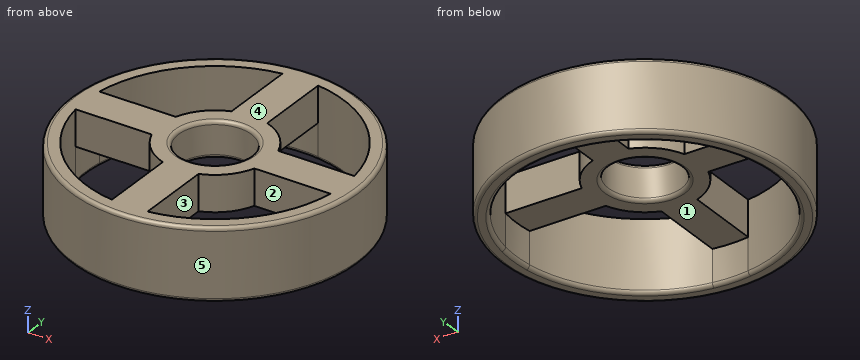
```python
from build123d import *

# Parameters (mm, degrees)
SKETCH2_R           = 20
BOSS_EXTRUDE1_DEPTH = 10
SKETCH4_R           = 5.1
CUT_EXTRUDE1_DEPTH  = 31
CUT_EXTRUDE2_START  = -5
SKETCH5_R           = 18
CUT_EXTRUDE2_DEPTH  = 5
FILLET1_R           = 0.5


with BuildPart() as part:
    # Sketch2 → Boss-Extrude1 (new body)
    with BuildSketch(Plane.XY):
        Circle(SKETCH2_R)
    extrude(amount=BOSS_EXTRUDE1_DEPTH)

    # Sketch4 → Cut-Extrude1 (cut, through all)
    with BuildSketch(Plane.XY.offset(10)):
        Circle(SKETCH4_R)
        with BuildLine():
            Line((-2.5, 17.82554347), (-2.5, 7.177046746))
            ThreePointArc((-2.5, 7.177046746), (-5.374011537, 5.374011537), (-7.177046746, 2.5))
            Line((-7.177046746, 2.5), (-17.82554347, 2.5))
            ThreePointArc((-17.82554347, 2.5), (-12.727922061, 12.727922061), (-2.5, 17.82554347))
        make_face()
        with BuildLine():
            Line((2.5, 17.82554347), (2.5, 7.177046746))
            ThreePointArc((2.5, 7.177046746), (5.374011537, 5.374011537), (7.177046746, 2.5))
            Line((7.177046746, 2.5), (17.82554347, 2.5))
            ThreePointArc((17.82554347, 2.5), (12.727922061, 12.727922061), (2.5, 17.82554347))
        make_face()
        with BuildLine():
            Line((7.177046746, -2.5), (17.82554347, -2.5))
            ThreePointArc((17.82554347, -2.5), (12.727922061, -12.727922061), (2.5, -17.82554347))
            Line((2.5, -17.82554347), (2.5, -7.177046746))
            ThreePointArc((2.5, -7.177046746), (5.374011537, -5.374011537), (7.177046746, -2.5))
        make_face()
        with BuildLine():
            Line((-7.177046746, -2.5), (-17.82554347, -2.5))
            ThreePointArc((-17.82554347, -2.5), (-12.727922061, -12.727922061), (-2.5, -17.82554347))
            Line((-2.5, -17.82554347), (-2.5, -7.177046746))
            ThreePointArc((-2.5, -7.177046746), (-5.374011537, -5.374011537), (-7.177046746, -2.5))
        make_face()
    extrude(amount=-CUT_EXTRUDE1_DEPTH, mode=Mode.SUBTRACT)

    # Sketch5 → Cut-Extrude2 (cut)
    with BuildSketch(Plane(origin=(0, 0, 0), x_dir=(-1, 0, 0), z_dir=(0, 0, -1)).offset(CUT_EXTRUDE2_START)):
        with Locations(Location((0, 0, 0), (0, 0, 172.016443854))):
            Circle(SKETCH5_R)
    extrude(amount=CUT_EXTRUDE2_DEPTH, mode=Mode.SUBTRACT)

    # Fillet1
    fillet1_edges = [part.edges().sort_by_distance(p)[0] for p in [
        (-20, 0, 0),
        (-18, 0, 0),
        (-5.1, 0, 10),
        (-20, 0, 10),
        (-5.1, 0, 5),
    ]]
    fillet(fillet1_edges, radius=FILLET1_R)


solid = part.part
```
Verification items for the finished model (mm, model axes). Face numbers are marked on the shaded views. A direction names the side the tool comes from. Coordinates: 2 decimals unless noted, no trailing zeros. Loops run counter-clockwise (first coordinate to the right, second up) from the corner with the lowest first, then second, coordinate; pieces in that order, holes last. Notation, with made-up numbers: (-33, 89) - (-4, 89) arc R35 ccw to (-4, 123) - close; hole circle Ø3 at (58, 61). An arc over 180 degrees is marked (long way). Return JSON: item names as keys, results as strings.
1. Section check A-A, the plane x = 0. Record the boundary of the cut face in (y, z).
Established:
{"outline": "(-20, 0.5) arc R0.5 ccw to (-19.5, 0) - (-18.5, 0) arc R0.5 ccw to (-18, 0.5) - (-18, 5) - (-5.6, 5) arc R0.5 ccw to (-5.1, 5.5) - (-5.1, 9.5) arc R0.5 ccw to (-5.6, 10) - (-19.5, 10) arc R0.5 ccw to (-20, 9.5) - close; (5.1, 5.5) arc R0.5 ccw to (5.6, 5) - (18, 5) - (18, 0.5) arc R0.5 ccw to (18.5, 0) - (19.5, 0) arc R0.5 ccw to (20, 0.5) - (20, 9.5) arc R0.5 ccw to (19.5, 10) - (5.6, 10) arc R0.5 ccw to (5.1, 9.5) - close"}
2. Go/stop test with flat-tipped pins: pin 1 (2.5 mm diameter, centred on x = 13, z = 8.5, fed in from +Y); pin 2 (6 mm diameter, centred on x = 10.5, z = 4, fed in from -Y); pin 3 (5.5 mm diameter, centred on y = 15, z = 7.5, fed in from -X); pin 4 (3 mm diameter, centred on x = 7.5, y = 7.5, fed in from -Z). Record where each tip stops, or that it passes through.
Established:
{"pin 1": "stops at y = 16.18", "pin 2": "stops at y = -18.54", "pin 3": "stops at x = -15.81", "pin 4": "passes through"}
3. Thickness scan on L1, parallel to Y at x = 0, z = 6.55; L2, parallel to X at y = 0.5, z = 4.75; L3, parallel to X at y = -6.5, z = 9.5. Record the ranges inside material, lowest first.
Established:
{"L1": "y = -20 to -5.1, 5.1 to 20", "L2": "x = -19.99 to -17.99, 17.99 to 19.99", "L3": "x = -18.91 to -16.79, -3.94 to 3.94, 16.79 to 18.91"}
4. Section check D-D, the plane y = -8.5. Count the separate pieces of the cut face and the enclosed holes in it, then the cut area to 3 significant figures.
Established:
{"separate pieces": "3", "enclosed holes": "0", "area": "69.4 mm2"}
5. Section check C-C, the plane z = 7. Record the boundary of the cut face in (x, y).
Established:
{"outline": "circle Ø40 at (0, 0); hole (-17.83, -2.5) arc R18 ccw to (-2.5, -17.83) - (-2.5, -7.18) arc R7.6 cw to (-7.18, -2.5) - close; hole (-17.83, 2.5) - (-7.18, 2.5) arc R7.6 cw to (-2.5, 7.18) - (-2.5, 17.83) arc R18 ccw to start; hole circle Ø10.2 at (0, 0); hole (2.5, -17.83) arc R18 ccw to (17.83, -2.5) - (7.18, -2.5) arc R7.6 cw to (2.5, -7.18) - close; hole (2.5, 7.18) arc R7.6 cw to (7.18, 2.5) - (17.83, 2.5) arc R18 ccw to (2.5, 17.83) - close"}
6. Tool access check on the marked faces 1 and 2. Record the directions out of +Z, -Z, +X, -X, +Y, -Y that give a thin tool (end or side, any length) a straight path to the whole face; none if there is none.
Established:
{"face 1": "-Z", "face 2": "+Z, -Z"}
7. Mould release check, pull along X, two halves, no side actions. Record for the marked faces 3, 4 and 5: +X half, -X half, draft (parallel to the pull), parting line (faces both ways), or undercut.
Established:
{"face 3": "undercut", "face 4": "draft", "face 5": "parting line"}
